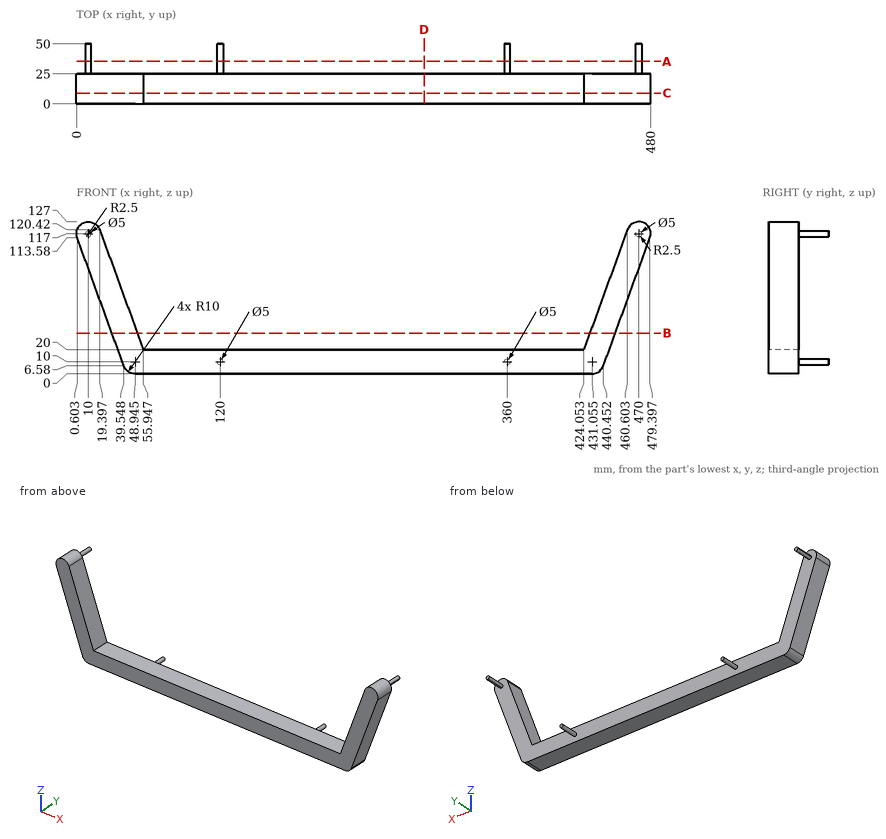
Input: dimensioned drawing with shaded views. Units: mm. Origin: part minimum x, y, z. Coordinates: 2 decimals unless noted, no trailing zeros. Loops run counter-clockwise (first coordinate to the right, second up) from the corner with the lowest first, then second, coordinate; pieces in that order, holes last. Notation, with made-up numbers: M 14,79 L 32,79 A32 cw 32,116 Z; hole C 37.5,-36.75 d11. An arc over 180 degrees is marked long. Use a Markdown table: item, result. Add a question column.
Q1. Section query A-A, the plane y = 35.5. Return loops of the section in (x, z) (1 decimal).
Q2. Section query B-B, the plane z = 34. Return loops of the section in (x, y).
Q3. First-contact query: pin 1 (3 mm diameter, centred on y = 21, z = 99, fed in from +X); pin 2 (12.5 mm diameter, centred on x = 271.5, y = 15.5, fed in from +Z). Flat tips, straight axial feed; report the tip coordinate or a pass-through.
Q4. Section query D-D, the plane x = 290.5. Return loops of the section in (y, z), and give its area (3 significant figures).
Q5. Material intervals for L1, parallel to Z at x = 101.5, y = 23; L2, parallel to X at y = 21, z = 23 (1 decimal); L3, parallel to Y at x = 102.5, z = 17, sorted ascending.
Q6. Section query C-C, the plane y = 9. Return loops of the section in (x, z) (1 decimal), and give its area (3 significant figures).
Result:
| question | item | result |
|---|---|---|
| 1 | outline | C 10,117 d5; C 120,10 d5; C 360,10 d5; C 470,117 d5 |
| 2 | outline | M 29.57,0 L 50.85,0 L 50.85,25 L 29.57,25 Z; M 429.15,0 L 450.43,0 L 450.43,25 L 429.15,25 Z |
| 3 | pin 1 | stops at x = 474.64 |
| 3 | pin 2 | stops at z = 20 |
| 4 | outline | M 0,0 L 25,0 L 25,20 L 0,20 Z |
| 4 | area | 500 mm2 |
| 5 | L1 | z = 0 to 20 |
| 5 | L2 | x = 33.6 to 54.9, 425.1 to 446.4 |
| 5 | L3 | y = 0 to 25 |
| 6 | outline | M 0.6,113.6 L 39.5,6.6 A10 ccw 48.9,0 L 431.1,0 A10 ccw 440.5,6.6 L 479.4,113.6 A10 ccw 460.6,120.4 L 424.1,20 L 55.9,20 L 19.4,120.4 A10 ccw Z |
| 6 | area | 12,500 mm2 |
